For this review, take the finished solid that the model builds, in its own axes (mm). A direction names the side the tool comes from. Round coordinates to 2 decimals unless told otherwise and drop trailing zeros. Write each loop counter-clockwise with the first axis right and the second up, starting at its lowest first coordinate (ties: lowest second). Pieces come first, ordered by that corner, then holes. Notation, with made-up numbers: (85.5, 8.5) -> (94.5, 8.5) arc R22 cw to (94.5, 30.5) -> close; hole circle Ø2 at (-14, 51.5). An arc over 180 degrees is marked (long way). Answer as CSV lines item,"result". Start each with the question number.
Item 1: Take a section at B-B on z = -7.5. Give the boundary of the cut face in (x, y).
Item 2: For pin 1 Ø3 at (x, z) = (2.5, -21) entering from -Y; pin 2 Ø1.5 at (y, z) = (-1.5, 0) entering from +X; pin 3 Ø0.7 at (x, z) = (0.5, 3) entering from +Y, all flat-tipped, find the tip position at first contact; note any pin that passes through.
Item 3: Wall thickness on probe 1 along Z at (x, y) = (1.5, 2); probe 2 along Z at (x, y) = (1.5, -0.75); probe 3 along X at (y, z) = (0.75, -10): over which ranges is each line inside the solid? List them lowest first. Write a range as from..to.
Item 4: Machinability: for faces 1 (the cylindrical face through (-0.314, -2.392, -13.477)), 2 (the flat face through (0, 0, -25.4)), 3 (the flat face through (1.71, -1.01, 3.64)), which of the approach directions +Z, -Z, +X, -X, +Y, -Y give a long, thin tool a straight path to every point of the face, cutting with its end or side? Answer none if there is none.
Solid Edge part; units mm, degrees
sketch "Sketch1" plane through (0, 0, 0) normal (0, 0, 1) x (1, 0, 0)
  circle A0 centre (0, 0) radius 3.9624
extrude "Protrusion1" add sketch "Sketch1" along normal blind 4.826
sketch "Sketch2" plane through (0, 0, 0) normal (0, 0, -1) x (1, 0, 0)
  circle A0 centre (0, 0) radius 2.413
extrude "Protrusion2" add sketch "Sketch2" along normal blind 25.4
sketch "Sketch3" plane through (0, 0, -25.4) normal (0, 0, -1) x (1, 0, 0)
  circle A0 centre (0, 0) radius 2.4127
extrude "Cutout1" cut sketch "Sketch3" against normal blind 23.8125 flip side to cut
chamfer "Chamfer_1" distance 0.3619 angle 45 1 edges at (-2.4127, 0, -25.4)
sketch "Sketch4" plane through (0, 0, 4.826) normal (0, 0, 1) x (1, 0, 0)
  line L0 (-1.1457, 1.9844) -> (1.1457, 1.9844)
  line L1 (2.2914, 0) -> (1.1457, 1.9844)
  line L2 (1.1457, -1.9844) -> (2.2914, 0)
  line L3 (-1.1457, -1.9844) -> (1.1457, -1.9844)
  line L4 (-2.2914, 0) -> (-1.1457, -1.9844)
  line L5 (-1.1457, 1.9844) -> (-2.2914, 0)
extrude "Cutout2" cut sketch "Sketch4" against normal blind 2.413
properties part number "24101594"
Output values:
1,outline,"circle Ø4.83 at (0, 0)"
2,pin 1,"stops at y = -2.2"
2,pin 2,"stops at x = 3.89"
2,pin 3,"stops at y = 3.96"
3,probe 1,"z = 0..4.83"
3,probe 2,"z = -25.4..2.41"
3,probe 3,"x = -2.29..2.29"
4,face 1,"-Z"
4,face 2,"-Z, +X, -X, +Y, -Y"
4,face 3,"+Z"
